from build123d import *

# Parameters (mm, degrees)
ESQUISSE1_W        = 25
ESQUISSE1_H        = 10
ESQUISSE1_R        = 2
BOSS_EXTRU_1_DEPTH = 5
CONG_1_R           = 3
CONG_2_R           = 3
CONG_3_R           = 3
CONG_4_R           = 3


with BuildPart() as part:
    # Esquisse1 → Boss.-Extru.1 (new body)
    # profile 1 of 2: a face of its own
    with BuildSketch(Plane.XY):
        Rectangle(ESQUISSE1_W, ESQUISSE1_H)
        with Locations((-7.5, 0)):
            Circle(ESQUISSE1_R, mode=Mode.SUBTRACT)
    # profile 2 of 2: a face of its own
    with BuildSketch(Plane.XY):
        with Locations((25, 0)):
            Rectangle(ESQUISSE1_W, ESQUISSE1_H)
        with Locations((32.5, 0)):
            Circle(ESQUISSE1_R, mode=Mode.SUBTRACT)
    extrude(amount=BOSS_EXTRU_1_DEPTH)

    # Congé1
    cong_1_edges = [part.edges().sort_by_distance(p)[0] for p in [
        (37.5, 5, 2.5),
    ]]
    fillet(cong_1_edges, radius=CONG_1_R)

    # Congé2
    cong_2_edges = [part.edges().sort_by_distance(p)[0] for p in [
        (37.5, -5, 2.5),
    ]]
    fillet(cong_2_edges, radius=CONG_2_R)

    # Congé3
    cong_3_edges = [part.edges().sort_by_distance(p)[0] for p in [
        (-12.5, 5, 2.5),
    ]]
    fillet(cong_3_edges, radius=CONG_3_R)

    # Congé4
    cong_4_edges = [part.edges().sort_by_distance(p)[0] for p in [
        (-12.5, -5, 2.5),
    ]]
    fillet(cong_4_edges, radius=CONG_4_R)


solid = part.part
Part model, mm, in its own coordinate system. Coordinates: 2 decimals unless noted, no trailing zeros. Loops run counter-clockwise (first coordinate to the right, second up) from the corner with the lowest first, then second, coordinate; pieces in that order, holes last. Notation, with made-up numbers: (89.5, -18.75) -> (141.5, -18.75) arc R20 ccw to (141.5, 18.25) -> close; hole circle Ø8 at (7.25, 71.5). An arc over 180 degrees is marked (long way). Use a Markdown table: item, result. Add a question column.
Item 1: Band-saw the part on C-C on y = 0. Write the cut outline in (x, z), plus the area to 3 significant figures.
Item 2: Band-saw the part on D-D on y = 3.75. Write the cut outline in (x, z), plus the area to 3 significant figures.
Item 3: Band-saw the part on A-A on x = 32.5. Write the cut outline in (y, z), plus the area to 3 significant figures.
Item 4: Probe probe 1 along Y at (x, z) = (32.5, 2.6); probe 2 along X at (y, z) = (-0.5, 3.45); probe 3 along X at (y, z) = (-0.25, 2.8). List the from-to ranges inside material, lowest first.
Item 5: Pull direction Y, two halves, no side cores. Call faces 1 (the flat face through (12, -5, 2)), 2 (the cylindrical face through (-9.498, 0.088, 2.465)), 3 (the flat face through (12, 0, 0)), 4 (the cylindrical face through (36.6, 4.14, 2.54)): +Y half, -Y half, draft (parallel to the pull), parting line (faces both ways), or undercut.
Item 6: Band-saw the part on B-B on z = 1.6. Write the cut outline in (x, y).
Geometry says:
| question | item | result |
|---|---|---|
| 1 | outline | (-12.5, 0) -> (-9.5, 0) -> (-9.5, 5) -> (-12.5, 5) -> close; (-5.5, 0) -> (30.5, 0) -> (30.5, 5) -> (-5.5, 5) -> close; (34.5, 0) -> (37.5, 0) -> (37.5, 5) -> (34.5, 5) -> close |
| 1 | area | 210 mm² |
| 2 | outline | (-11.94, 0) -> (36.94, 0) -> (36.94, 5) -> (-11.94, 5) -> close |
| 2 | area | 244 mm² |
| 3 | outline | (-5, 0) -> (-2, 0) -> (-2, 5) -> (-5, 5) -> close; (2, 0) -> (5, 0) -> (5, 5) -> (2, 5) -> close |
| 3 | area | 30.0 mm² |
| 4 | probe 1 | -5 to -2, 2 to 5 |
| 4 | probe 2 | -12.5 to -9.44, -5.56 to 30.56, 34.44 to 37.5 |
| 4 | probe 3 | -12.5 to -9.48, -5.52 to 30.52, 34.48 to 37.5 |
| 5 | face 1 | -Y half |
| 5 | face 2 | undercut |
| 5 | face 3 | draft |
| 5 | face 4 | +Y half |
| 6 | outline | (-12.5, -2) arc R3 ccw to (-9.5, -5) -> (34.5, -5) arc R3 ccw to (37.5, -2) -> (37.5, 2) arc R3 ccw to (34.5, 5) -> (-9.5, 5) arc R3 ccw to (-12.5, 2) -> close; hole circle Ø4 at (-7.5, 0); hole circle Ø4 at (32.5, 0) |
